from build123d import *

# Parameters (mm, degrees)
EXTRUDE_THIN1_DEPTH = 793.75
FILLET1_R           = 1.143


with BuildPart() as part:
    # Sketch1 → Extrude-Thin1 (new body)
    with BuildSketch(Plane.XY):
        with BuildLine():
            Line((0, 0), (-26.9875, 0))
            Line((-26.9875, 0), (-26.9875, 36.5125))
            Line((-26.9875, 36.5125), (-30.1625, 36.5125))
            Line((-30.1625, 36.5125), (-30.1625, 49.312109381))
            ThreePointArc((-30.1625, 49.312109381), (-33.3375, 57.712369794), (-41.275, 61.9125))
            Line((-41.275, 61.9125), (-41.275, 79.375))
            Line((-41.275, 79.375), (-10.31875, 79.375))
            Line((-10.31875, 79.375), (-10.31875, 78.232))
            Line((-10.31875, 78.232), (-40.132, 78.232))
            Line((-40.132, 78.232), (-40.132, 62.883145405))
            ThreePointArc((-40.132, 62.883145405), (-32.152062089, 58.082238727), (-29.0195, 49.312109381))
            Line((-29.0195, 49.312109381), (-29.0195, 37.6555))
            Line((-29.0195, 37.6555), (-25.8445, 37.6555))
            Line((-25.8445, 37.6555), (-25.8445, 1.143))
            Line((-25.8445, 1.143), (0, 1.143))
            Line((0, 1.143), (0, 0))
        make_face()
    extrude(amount=-EXTRUDE_THIN1_DEPTH)

    # Fillet1
    fillet1_edges = [part.edges().sort_by_distance(p)[0] for p in [
        (-25.8445, 37.6555, -396.875),
        (-26.9875, 0, -396.875),
        (-30.1625, 36.5125, -396.875),
        (-41.275, 61.9125, -396.875),
        (-41.275, 79.375, -396.875),
    ]]
    fillet(fillet1_edges, radius=FILLET1_R)


solid = part.part
Verification items for the finished model (mm, model axes). A direction names the side the tool comes from. Give positions to 0.01 mm unless a question says otherwise; leave off trailing zeros. Write each loop counter-clockwise with the first axis right and the second up, starting at its lowest first coordinate (ties: lowest second). Pieces come first, ordered by that corner, then holes. Notation, with made-up numbers: (51.5, 3.25) - (102.5, 3.25) arc R7 ccw to (102.5, 7.25) - close; hole circle Ø10 at (-29.75, 25). An arc over 180 degrees is marked (long way). Answer as CSV lines item,"result". Start each with the question number.
1. Sectioned sample at A-A (z = -556). Record the boundary of the cut face in (x, y) (1 decimal).
2. Thickness scan on line 1 (Y direction, x = -28, z = -351) (1 decimal); line 2 (Y direction, x = -14.5, z = -354.5) (3 decimals); line 3 (X direction, y = 32.5, z = -326). Record the ranges inside material, lowest first.
3. Depth check by flat-ended pin: pin 1 (3 mm diameter, centred on y = 24.5, z = -604.5, fed in from +X); pin 2 (10.5 mm diameter, centred on y = 23, z = -304, fed in from -X); pin 3 (5 mm diameter, centred on x = -24.5, y = 23, fed in from +Z); pin 4 (0.6 mm diameter, centred on x = -28.5, z = -486.5, fed in from -Y). Enter the tip coordinate at first touch or a pass-through.
4. Set-up check for faces 1 (the face through (-26.988, 19, -391)), 2 (the face through (-25.844, 19, -391)), 3 (the face through (-30, 40, -793.75)): record each of +Z, -Z, +X, -X, +Y, -Y from which the full face is reachable in a straight line by a thin tool's end or side.
5. Sectioned sample at B-B (y = 21). Record the boundary of the cut face in (x, z), then the cut area to 3 significant figures.
6. Draft check along Y on faces 4 (the face through (-32.237, 58.185, -391.319)), 5 (the face through (-40.132, 71, -391)), 6 (the face through (-41.275, 70, -391)), 7 (the face through (-13, 0, -391)). Enter one of: pulls with the +Y half, pulls with the -Y half, needs draft (parallel to the pull), parting line crosses it, or undercut.
Derived:
1,outline,"(-41.3, 62.9) arc R1.1 ccw to (-40.4, 61.8) arc R12.7 cw to (-30.2, 49.3) - (-30.2, 37.7) arc R1.1 ccw to (-29, 36.5) - (-27, 36.5) - (-27, 1.1) arc R1.1 ccw to (-25.8, 0) - (0, 0) - (0, 1.1) - (-25.8, 1.1) - (-25.8, 36.5) arc R1.1 ccw to (-27, 37.7) - (-29, 37.7) - (-29, 49.3) arc R13.8 ccw to (-40.1, 62.9) - (-40.1, 78.2) - (-10.3, 78.2) - (-10.3, 79.4) - (-40.1, 79.4) arc R1.1 ccw to (-41.3, 78.2) - close"
2,line 1,"36.5 to 37.7, 78.2 to 79.4"
2,line 2,"0 to 1.143, 78.232 to 79.375"
2,line 3,"-26.99 to -25.84"
3,pin 1,"x = -25.84"
3,pin 2,"x = -26.99"
3,pin 3,"z = 0"
3,pin 4,"y = 36.51"
4,face 1,"+Z, -Z, -X, -Y"
4,face 2,"+Z, -Z, +X"
4,face 3,"-Z, +X, -X, +Y, -Y"
5,outline,"(-26.99, -793.75) - (-25.84, -793.75) - (-25.84, 0) - (-26.99, 0) - close"
5,area,"907 mm²"
6,face 4,"undercut"
6,face 5,"undercut"
6,face 6,"needs draft"
6,face 7,"pulls with the -Y half"
